from build123d import *

# Parameters (mm, degrees)
SKETCH_1_W               = 154
SKETCH_1_H               = 154
EXTRUDE_1_DEPTH          = 7
SKETCH_7_W               = 10.6
SKETCH_7_H               = 5.6
CUT_EXTRUDE_2_DEPTH      = 2
SKETCH_8_W               = 115
SKETCH_8_H               = 115
CUT_EXTRUDE_3_DEPTH      = 110.119200877
SKETCH_11_W              = 20
SKETCH_11_H              = 7
EXTRUDE_6_DEPTH          = 15
MIRROR_6_COPY_1_SKETCH_W = 20
MIRROR_6_COPY_1_SKETCH_H = 7
MIRROR_6_COPY_1_DEPTH    = 15
FILLET_6_R               = 2
CHAMFER_5_SIZE           = 2
HOLE_WIZARD_M31_D        = 3.15
SKETCH_14_R              = 2.15
CUT_EXTRUDE_4_DEPTH      = 5


with BuildPart() as part:
    # Эскиз1 → Бобышка-Вытянуть1 (new body)
    with BuildSketch(Plane(origin=(0, 0, 0), x_dir=(1, 0, 0), z_dir=(0, 1, 0))):
        Rectangle(SKETCH_1_W, SKETCH_1_H)
    extrude(amount=EXTRUDE_1_DEPTH)

    # Эскиз7 → Вырез-Вытянуть2 (cut)
    with BuildSketch(Plane.XZ):
        with Locations((-67.25, 67.25)):
            Rectangle(SKETCH_7_W, SKETCH_7_H)
        with Locations((67.25, 67.25)):
            Rectangle(SKETCH_7_W, SKETCH_7_H)
        with Locations((-67.25, -67.25)):
            Rectangle(SKETCH_7_W, SKETCH_7_H)
        with Locations((67.25, -67.25)):
            Rectangle(SKETCH_7_W, SKETCH_7_H)
    extrude(amount=-CUT_EXTRUDE_2_DEPTH, mode=Mode.SUBTRACT)

    # Эскиз8 → Вырез-Вытянуть3 (cut, through all)
    with BuildSketch(Plane(origin=(0, 7, 0), x_dir=(1, 0, 0), z_dir=(0, 1, 0))):
        Rectangle(SKETCH_8_W, SKETCH_8_H)
    extrude(amount=-CUT_EXTRUDE_3_DEPTH, mode=Mode.SUBTRACT)

    # Эскиз11 → Бобышка-Вытянуть6 (add)
    with BuildSketch(Plane(origin=(77, 0, 0), x_dir=(0, 0, -1), z_dir=(1, 0, 0))):
        with Locations((-67, 3.5)):
            Rectangle(SKETCH_11_W, SKETCH_11_H)
    extrude_6 = extrude(amount=EXTRUDE_6_DEPTH)

    # Зеркальное отражение5: Бобышка-Вытянуть6 across plane
    add(extrude_6.mirror(Plane.XY))

    # Зеркальное отражение6: Бобышка-Вытянуть6 across plane
    add(extrude_6.mirror(Plane(origin=(0, 0, 0), x_dir=(0, 0, 1), z_dir=(1, 0, 0))))

    # Зеркальное отражение6 copy 1 sketch → Зеркальное отражение6 copy 1 (add)
    with BuildSketch(Plane.ZY.offset(77)):
        with Locations((-67, 3.5)):
            Rectangle(MIRROR_6_COPY_1_SKETCH_W, MIRROR_6_COPY_1_SKETCH_H)
    extrude(amount=MIRROR_6_COPY_1_DEPTH)

    # Скругление6
    fillet_6_edges = [part.edges().sort_by_distance(p)[0] for p in [
        (57.5, 3.5, -57.5),
        (57.5, 3.5, 57.5),
        (-57.5, 3.5, 57.5),
        (-57.5, 3.5, -57.5),
    ]]
    fillet(fillet_6_edges, radius=FILLET_6_R)

    # Chamfer 5
    chamfer_5_edges = [part.edges().sort_by_distance(p)[0] for p in [
        (-92, 3.5, 77),
        (-92, 7, 67),
        (-92, 3.5, 57),
        (-84.5, 7, 57),
        (-77, 7, 0),
        (-84.5, 7, -57),
        (-92, 3.5, -57),
        (-92, 7, -67),
        (-92, 3.5, -77),
        (0, 7, -57.5),
        (57.5, 7, 0),
        (0, 7, 57.5),
        (-57.5, 7, 0),
        (56.914213562, 7, -56.914213562),
        (56.914213562, 7, 56.914213562),
        (-56.914213562, 7, -56.914213562),
        (-56.914213562, 7, 56.914213562),
        (0, 7, 77),
        (77, 7, 0),
        (84.5, 7, 57),
        (92, 3.5, 57),
        (92, 7, 67),
        (92, 3.5, 77),
        (0, 7, -77),
        (92, 3.5, -77),
        (92, 7, -67),
        (92, 3.5, -57),
        (84.5, 7, -57),
    ]]
    chamfer(chamfer_5_edges, length=CHAMFER_5_SIZE)

    # Сверло под метчик  спиральное M31 (through all)
    with Locations(Plane(origin=(0, 7, 0), x_dir=(1, 0, 0), z_dir=(0, 1, 0))):
        with Locations((82.5, -67), (-82.5, 67), (82.5, 67), (-82.5, -67)):
            Hole(HOLE_WIZARD_M31_D / 2)

    # Эскиз14 → Вырез-Вытянуть4 (cut)
    with BuildSketch(Plane(origin=(0, 7, 0), x_dir=(1, 0, 0), z_dir=(0, 1, 0))):
        with Locations(Location((-82.5, 67, 0), (0, 0, 270))):
            Circle(SKETCH_14_R)
        with Locations(Location((82.5, 67, 0), (0, 0, 270))):
            Circle(SKETCH_14_R)
        with Locations(Location((-82.5, -67, 0), (0, 0, 270))):
            Circle(SKETCH_14_R)
        with Locations(Location((82.5, -67, 0), (0, 0, 270))):
            Circle(SKETCH_14_R)
    extrude(amount=-CUT_EXTRUDE_4_DEPTH, mode=Mode.SUBTRACT)


solid = part.part
Model file for the job. Use its own axes, mm. A direction names the side the tool comes from. Give positions to 0.01 mm unless a question says otherwise; leave off trailing zeros. Write each loop counter-clockwise with the first axis right and the second up, starting at its lowest first coordinate (ties: lowest second). Pieces come first, ordered by that corner, then holes. Notation, with made-up numbers: (35.25, 42) -> (42.25, 42) arc R25 cw to (42.25, 67) -> close; hole circle Ø2 at (61.25, 1). An arc over 180 degrees is marked (long way). Write item = value, one per line.
(1) Slice it at B-B, the plane z = 53. Give the cut face in (x, y).
Determined:
outline = (-77, 0) -> (-57.5, 0) -> (-57.5, 5) -> (-59.5, 7) -> (-75, 7) -> (-77, 5) -> close; (57.5, 0) -> (77, 0) -> (77, 5) -> (75, 7) -> (59.5, 7) -> (57.5, 5) -> close
(2) Slice it at A-A, the plane x = -29. Give the cut face in (y, z).
Determined:
outline = (0, -77) -> (5, -77) -> (7, -75) -> (7, -59.5) -> (5, -57.5) -> (0, -57.5) -> close; (0, 57.5) -> (5, 57.5) -> (7, 59.5) -> (7, 75) -> (5, 77) -> (0, 77) -> close
(3) Flat gauge pins, fed straight in: P1, Ø1.5, axis at y = 3.5, z = -10.5, coming from the -X side; P2, Ø1.3, axis at x = -82, z = -66, coming from the +Y side; P3, Ø1.5, axis at y = 1.5, z = -3.5, coming from the +X side. Where does each tip first touch, or does it go through?
Determined:
P1 = -77
P2 = 2
P3 = 77
(4) Slice it at C-C, the plane x = 70.5. Give the cut face in (y, z).
Determined:
outline = (0, -77) -> (5, -77) -> (7, -75) -> (7, 75) -> (5, 77) -> (0, 77) -> (0, 70.05) -> (2, 70.05) -> (2, 64.45) -> (0, 64.45) -> (0, -64.45) -> (2, -64.45) -> (2, -70.05) -> (0, -70.05) -> close
(5) Probe line 1 along X through (y, z) = (3.85, -67); line 2 along Z through (x, y) = (-82.5, 1.05) (3 decimals); line 3 along Z through (x, y) = (43, 1.5). List the from-to ranges inside material, lowest first.
Determined:
line_1 = -92 to -84.65, -80.35 to 80.35, 84.65 to 92
line_2 = -77 to -68.575, -65.425 to -57, 57 to 65.425, 68.575 to 77
line_3 = -77 to -57.5, 57.5 to 77
(6) Mould opens along Z. For faces 5 (the face through (-60, 7, 11)), 6 (the face through (57.496, 5.792, 57.452)) say: released by +Z, released by -Z, zero draft, split by the parting line, or undercut.
Determined:
face_5 = zero draft
face_6 = undercut
(7) Tool access for faces 1 (the face through (80.4, 4.54, 66.53)), 2 (the face through (-1, 3, -57.5)), 3 (the face through (-77, 2, 1)), 4 (the face through (83, 2, -57)): list every direction of +Z, -Z, +X, -X, +Y, -Y with a clear straight run to the whole face (end or side of a thin tool).
Determined:
face_1 = +Y
face_2 = +Y, -Y
face_3 = -X, +Y, -Y
face_4 = +X, +Y, -Y
